For this review, take the finished solid that the model builds, in its own axes (mm). Face numbers are marked on the shaded views. A direction names the side the tool comes from. Round coordinates to 2 decimals unless told otherwise and drop trailing zeros. Loops run counter-clockwise (first coordinate to the right, second up) from the corner with the lowest first, then second, coordinate; pieces in that order, holes last. Notation, with made-up numbers: (48, 15) -> (100, 15) arc R24 cw to (100, 34) -> close; hole circle Ø10 at (14.5, 45). An arc over 180 degrees is marked (long way). One line per question, with ' | ' between items. Start each with the question number.
1. Consider section B-B (x = 3). Write out the cut boundary in (y, z), and give its area (3 significant figures).
2. For pin 1 Ø1.9 at (x, z) = (17.5, -12) entering from -Y; pin 2 Ø5.5 at (x, y) = (-7, -43) entering from -Z, all flat-tipped, find the tip position at first contact; note any pin that passes through.
3. Draft analysis for pull direction Y (two halves, no side actions). For the marked faces 4, 5 and 6, state which applies: pulls with the +Y half, pulls with the -Y half, needs draft (parallel to the pull), parting line crosses it, or undercut.
4. Consider section A-A (z = -10.25). Write out the cut boundary in (x, y).
5. For the marked faces 1, 2 and 3, list the 3-axis set-ups (+Z, -Z, +X, -X, +Y, -Y) from which the entire face can be reached by the end or side of a thin tool; tool diameter is ignored.
6. Consider section C-C (y = -1.5). Write out the cut boundary in (x, z).
7. Consider section D-D (y = -33). Write out the cut boundary in (x, z).
8. Wall thickness on line 1 along Y through (x, z) = (-15, 1); line 2 along X through (y, z) = (-12.5, -13.75); line 3 along Z through (x, y) = (-13, -40.5): over which ranges is each line inside the solid? List them lowest first.
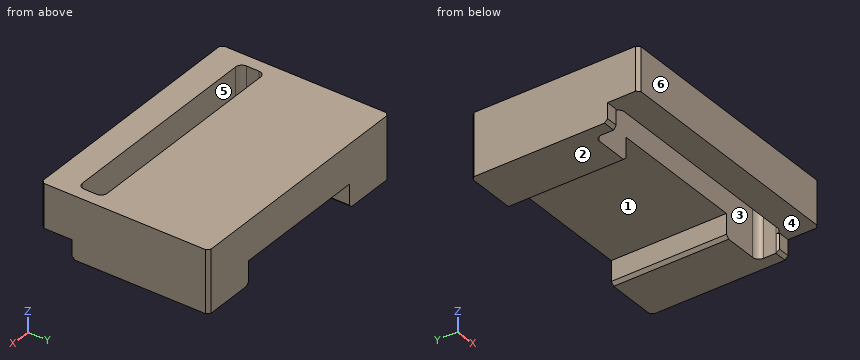
```python
from build123d import *

# Parameters (mm, degrees)
BOSS_EXTRUDE1_DEPTH      = 5
BOSS_EXTRUDE1_DEPTH_BACK = 15
SKETCH1_W                = 79
SKETCH1_H                = 54
SKETCH3_W                = 79
SKETCH3_H                = 10
CUT_EXTRUDE1_DEPTH       = 1
SKETCH4_W                = 71
SKETCH4_H                = 8
CUT_EXTRUDE2_DEPTH       = 15
SKETCH5_W                = 44
SKETCH5_H                = 35
CUT_EXTRUDE3_DEPTH       = 2.5
SKETCH6_W                = 44
SKETCH6_H                = 2.5
CUT_EXTRUDE4_DEPTH       = 80.907759323
SKETCH7_W                = 71
SKETCH7_H                = 8
CUT_EXTRUDE5_DEPTH       = 80.285875161
SKETCH8_W                = 44
SKETCH8_H                = 37
CUT_EXTRUDE6_DEPTH       = 5
CUT_EXTRUDE7_DEPTH       = 5
FILLET1_R                = 2
CHAMFER2_SIZE            = 1
CHAMFER3_SIZE            = 1
CHAMFER4_SIZE            = 1


with BuildPart() as part:
    # Sketch1 → Boss-Extrude1 (new, two sides: drawn at the far end of the back side and taken through both)
    with BuildSketch(Plane.XY.offset(-BOSS_EXTRUDE1_DEPTH_BACK)):
        with Locations((-21, -22)):
            Rectangle(SKETCH1_W, SKETCH1_H)
    extrude(amount=BOSS_EXTRUDE1_DEPTH + BOSS_EXTRUDE1_DEPTH_BACK)

    # Sketch3 → Cut-Extrude1 (cut)
    with BuildSketch(Plane(origin=(0, 0, -15), x_dir=(-1, 0, 0), z_dir=(0, 0, -1))):
        with Locations((21, -44)):
            Rectangle(SKETCH3_W, SKETCH3_H)
    extrude(amount=-CUT_EXTRUDE1_DEPTH, mode=Mode.SUBTRACT)

    # Sketch4 → Cut-Extrude2 (cut)
    with BuildSketch(Plane(origin=(0, 0, -15), x_dir=(-1, 0, 0), z_dir=(0, 0, -1))):
        with Locations((21, -36)):
            Rectangle(SKETCH4_W, SKETCH4_H)
    extrude(amount=-CUT_EXTRUDE2_DEPTH, mode=Mode.SUBTRACT)

    # Sketch5 → Cut-Extrude3 (cut)
    with BuildSketch(Plane(origin=(0, 0, -15), x_dir=(-1, 0, 0), z_dir=(0, 0, -1))):
        with Locations((21, -16.5)):
            Rectangle(SKETCH5_W, SKETCH5_H)
    extrude(amount=-CUT_EXTRUDE3_DEPTH, mode=Mode.SUBTRACT)

    # Sketch6 → Cut-Extrude4 (cut, through all)
    with BuildSketch(Plane.XZ.offset(-1)):
        with Locations((-21, -13.75)):
            Rectangle(SKETCH6_W, SKETCH6_H)
    extrude(amount=-CUT_EXTRUDE4_DEPTH, mode=Mode.SUBTRACT)

    # Sketch7 → Cut-Extrude5 (cut, through all)
    with BuildSketch(Plane(origin=(0, 0, 0), x_dir=(-1, 0, 0), z_dir=(0, 0, -1))):
        with Locations((21, -36)):
            Rectangle(SKETCH7_W, SKETCH7_H)
    extrude(amount=-CUT_EXTRUDE5_DEPTH, mode=Mode.SUBTRACT)

    # Sketch8 → Cut-Extrude6 (cut)
    with BuildSketch(Plane(origin=(0, 0, -12.5), x_dir=(-1, 0, 0), z_dir=(0, 0, -1))):
        with Locations((21, -13.5)):
            Rectangle(SKETCH8_W, SKETCH8_H)
    extrude(amount=-CUT_EXTRUDE6_DEPTH, mode=Mode.SUBTRACT)

    # Sketch9 → Cut-Extrude7 (cut)
    with BuildSketch(Plane(origin=(0, 0, -14), x_dir=(-1, 0, 0), z_dir=(0, 0, -1))):
        Polygon((56.5, -40), (-14.5, -40), (-14.5, -39), (-18.5, -39), (-18.5, -49), (60.5, -49), (60.5, -39), (56.5, -39), align=None)
    extrude(amount=-CUT_EXTRUDE7_DEPTH, mode=Mode.SUBTRACT)

    # Fillet1
    fillet1_edges = [part.edges().sort_by_distance(p)[0] for p in [
        (14.5, -40, -2),
        (14.5, -32, -5),
        (-56.5, -32, -5),
        (-56.5, -40, -2),
    ]]
    fillet(fillet1_edges, radius=FILLET1_R)

    # Chamfer1
    # the kernel refuses this chamfer: 1, 0.732050808 mm, written as the material it takes off along each edge
    with BuildSketch(Plane(origin=(14.232050808, -39, -9), x_dir=(0.9974998388550008, -0.07066874474792476, 0), z_dir=(0, 0, -1))) as chamfer1_piece_1:
        with BuildLine():
            Line((0.534510572, 0), (0.183539981, -0.816493036))
            Line((0.183539981, -0.816493036), (0.163562724, -0.817446573))
            ThreePointArc((0.163562724, -0.817446573), (0.12384643, -0.40032394), (-0.017983891, -0.00875098))
            Line((-0.017983891, -0.00875098), (0.001413375, 0.019949997))
            ThreePointArc((0.001413375, 0.019949997), (0.267333969, 0.001110621), (0.535923947, 0.019949997))
            Line((0.535923947, 0.019949997), (0.534510572, 0))
        make_face()
    extrude(amount=8.092169631, mode=Mode.SUBTRACT)
    with BuildSketch(Plane(origin=(-56.232050808, -39, -17.092169631), x_dir=(-0.2877176347633081, 0.9577152826629675, 0), z_dir=(0, 0, 1))) as chamfer1_piece_2:
        with BuildLine():
            Line((0.836867853, 0), (0.11722766, 0.521497102))
            Line((0.11722766, 0.521497102), (0.098073354, 0.527251455))
            ThreePointArc((0.098073354, 0.527251455), (0.057547506, 0.261068897), (-0.019154306, 0.005754353))
            Line((-0.019154306, 0.005754353), (0.004593737, -0.019465292))
            ThreePointArc((0.004593737, -0.019465292), (0.417739168, 0.033033052), (0.833416807, -0.019700007))
            Line((0.833416807, -0.019700007), (0.836867853, 0))
        make_face()
    extrude(amount=8.092169631, mode=Mode.SUBTRACT)

    # Chamfer2
    chamfer2_edges = [part.edges().sort_by_distance(p)[0] for p in [
        (1, -13.5, -15),
        (-43, -13.5, -15),
    ]]
    chamfer(chamfer2_edges, length=CHAMFER2_SIZE)

    # Chamfer3
    chamfer3_edges = [part.edges().sort_by_distance(p)[0] for p in [
        (18.5, -49, -2),
        (-60.5, -49, -2),
        (-60.5, 5, -5),
        (18.5, 5, -5),
    ]]
    chamfer(chamfer3_edges, length=CHAMFER3_SIZE)

    # Chamfer4
    chamfer4_edges = [part.edges().sort_by_distance(p)[0] for p in [
        (-58.626032501, -39, -15),
        (16.626032501, -39, -15),
    ]]
    chamfer(chamfer4_edges, length=CHAMFER4_SIZE)


solid = part.part
```
Answer block:
1) outline: (-49, -9) -> (-40, -9) -> (-40, 5) -> (-49, 5) -> close; (-32, -15) -> (5, -15) -> (5, 5) -> (-32, 5) -> close | area: 866 mm2
2) pin 1: stops at y = -39 | pin 2: stops at z = -9
3) face 4: needs draft | face 5: undercut | face 6: pulls with the -Y half
4) outline: (-60.5, -39) -> (-56.75, -39) -> (-56.49, -38.24) arc R2 cw to (-56.5, -38) -> (-56.5, -34) arc R2 cw to (-54.5, -32) -> (-43, -32) -> (-43, 5) -> (-59.5, 5) -> (-60.5, 4) -> close; (1, -32) -> (12.5, -32) arc R2 cw to (14.5, -34) -> (14.5, -38) arc R2 cw to (14.49, -38.24) -> (14.75, -39) -> (18.5, -39) -> (18.5, 4) -> (17.5, 5) -> (1, 5) -> close
5) face 1: -Z, +Y | face 2: -Z, +X, -X, +Y, -Y | face 3: +Z, -Z
6) outline: (-60.5, -15) -> (-44, -15) -> (-43, -14) -> (-43, -7.5) -> (1, -7.5) -> (1, -14) -> (2, -15) -> (18.5, -15) -> (18.5, 5) -> (-60.5, 5) -> close
7) outline: (-60.5, -15) -> (-56.23, -15) -> (-56.23, 5) -> (-60.5, 5) -> close; (14.23, -15) -> (18.5, -15) -> (18.5, 5) -> (14.23, 5) -> close
8) line 1: y = -49 to -40, -32 to 5 | line 2: x = -60.5 to -43, 1 to 18.5 | line 3: z = -9 to 5
